Can you work these out from the model? Positions are in its coordinate system, mm. A direction names the side the tool comes from. Coordinates: 2 decimals unless noted, no trailing zeros. Order: outer loops, then holes, each group sorted by start corner. A loop starts at its lowest first (then second) coordinate and runs counter-clockwise, first axis right, second up. Notation, with made-up numbers: (47.25, 14) -> (71.25, 14) arc R10 ccw to (71.25, 33) -> close; hole circle Ø2 at (-8.75, 63.25). An arc over 180 degrees is marked (long way). Answer in a Markdown table with one row per item.
```python
from build123d import *

# Parameters (mm, degrees)
F0_R     = 1
F1_DEPTH = 2
F2_W     = 12
F2_H     = 8.5
F3_DEPTH = 8
F4_R     = 1.25
F5_DEPTH = 12.7


with BuildPart() as f1:
    # F0 (on Top) → F1 (new body)
    with BuildSketch(Plane.XY):
        with BuildLine():
            ThreePointArc((-10.308361, -2.149295), (-9.063565, -5.154499), (-6.058361, -6.399295))
            Line((-6.058361, -6.399295), (12.041639, -6.399295))
            ThreePointArc((12.041639, -6.399295), (15.046843, -5.154499), (16.291639, -2.149295))
            ThreePointArc((16.291639, -2.149295), (15.046843, 0.855909), (12.041639, 2.100705))
            Line((12.041639, 2.100705), (-6.058361, 2.100705))
            ThreePointArc((-6.058361, 2.100705), (-9.063565, 0.855909), (-10.308361, -2.149295))
        make_face()
        with Locations((-6.058361, -2.149295)):
            Circle(F0_R, mode=Mode.SUBTRACT)
        with Locations((12.041639, -2.149295)):
            Circle(F0_R, mode=Mode.SUBTRACT)
    extrude(amount=F1_DEPTH)

    # F2 (on face) → F3 (join)
    with BuildSketch(Plane.XY.offset(2)):
        with Locations((2.991639, -2.149295)):
            Rectangle(F2_W, F2_H)
    extrude(amount=F3_DEPTH)

    # F4 (on face) → F5 (join)
    with BuildSketch(Plane(origin=(0, 2.100705, 0), x_dir=(-1, 0, 0), z_dir=(0, 1, 0))):
        with Locations((-2.991639, 5)):
            Circle(F4_R)
    extrude(amount=F5_DEPTH)


solid = f1.part
```
(1) On a 3-axis mill with a long thin cutter (end or side, diameter ignored), from which of +Z, -Z, +X, -X, +Y, -Y can I reach the whole of each face in a straight line? I mean faces 1 (the flat face through (3, 14.801, 5)), 2 (the flat face through (8.992, -2, 6)), 3 (the flat face through (-3.008, -2, 6)). Say none if no direction works.
Response values:
| item | result |
|---|---|
| face 1 | +Z, -Z, +X, -X, +Y |
| face 2 | +Z, +X, +Y, -Y |
| face 3 | +Z, -X, +Y, -Y |
(2) We'd pull the mould along Y, two halves only. Please class faces 4 (the cylindrical face through (-7.057, -2.105, 0.986)), 5 (the cylindrical face through (3.26, 8.36, 3.78)), 6 (the cylindrical face through (11.043, -2.105, 0.986)), 7 (the flat face through (3, -6.399, 5)): +Y half, -Y half, draft (parallel to the pull), parting line (faces both ways), or undercut.
Response values:
| item | result |
|---|---|
| face 4 | undercut |
| face 5 | draft |
| face 6 | undercut |
| face 7 | -Y half |
(3) I need wall thicknesses on line 1 (Y direction, x = 9.75, z = 1.25); line 2 (X direction, y = -4, z = 6.25); line 3 (Z direction, x = 3, y = 4). Which ranges of each line are inside material? Lowest first, please. Write a range as [from, to].
Response values:
| item | result |
|---|---|
| line 1 | [-6.4, 2.1] |
| line 2 | [-3.01, 8.99] |
| line 3 | [3.75, 6.25] |
(4) Suppose I cut it at C-C (x = 5.25). Please give me the cut outline in (y, z).
Response values:
| item | result |
|---|---|
| outline | (-6.4, 0) -> (2.1, 0) -> (2.1, 10) -> (-6.4, 10) -> close |
(5) Suppose I cut it at D-D (y = 10.5). Please give me the cut outline in (x, z), and give its area (3 significant figures).
Response values:
| item | result |
|---|---|
| outline | circle Ø2.5 at (2.99, 5) |
| area | 4.91 mm2 |
(6) Suppose I cut it at A-A (z = 5). Please give me the cut outline in (x, y).
Response values:
| item | result |
|---|---|
| outline | (-3.01, -6.4) -> (8.99, -6.4) -> (8.99, 2.1) -> (4.24, 2.1) -> (4.24, 14.8) -> (1.74, 14.8) -> (1.74, 2.1) -> (-3.01, 2.1) -> close |
(7) Suppose I cut it at B-B (y = -4.5). Please give me the cut outline in (x, z).
Response values:
| item | result |
|---|---|
| outline | (-9.6, 0) -> (15.58, 0) -> (15.58, 2) -> (8.99, 2) -> (8.99, 10) -> (-3.01, 10) -> (-3.01, 2) -> (-9.6, 2) -> close |
(8) Will these pins go through, and if not, where does the flat tip stop? pin 1 Ø1.6 at (x, y) = (12.04, -2.15) entering from +Z; pin 2 Ø1.5 at (y, z) = (5.5, 4.5) entering from +X; pin 3 Ø1 at (x, z) = (5, 8) entering from +Y; pin 4 Ø6 at (x, y) = (14, 0) entering from +Z.
Response values:
| item | result |
|---|---|
| pin 1 | through |
| pin 2 | x = 4.24 |
| pin 3 | y = 2.1 |
| pin 4 | z = 2 |
